Geometry check sheet. Reference: the model listing, model coordinates, mm. Coordinates: 2 decimals unless noted, no trailing zeros. Loops run counter-clockwise (first coordinate to the right, second up) from the corner with the lowest first, then second, coordinate; pieces in that order, holes last. Notation, with made-up numbers: M 61.25,89.25 L 78.25,89.25 A18 ccw 78.25,107.25 Z; hole C 29.5,40 d11. An arc over 180 degrees is marked long. Use CSV: the item, a comma, the result in double quotes.
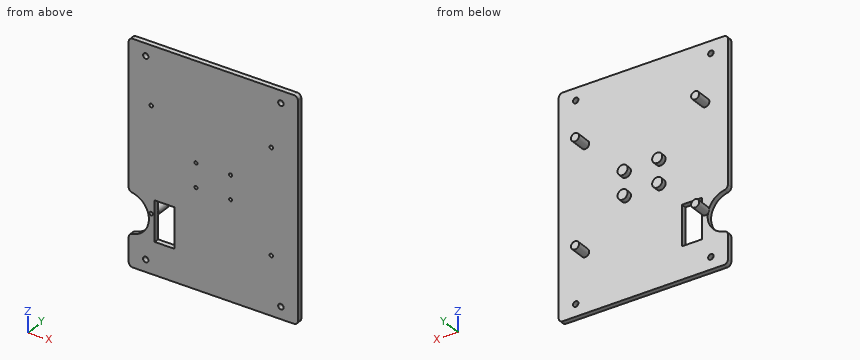
```python
from build123d import *

# Parameters (mm, degrees)
SKETCH1_W           = 107.315
SKETCH1_H           = 139.7
SKETCH1_R           = 1.7272
BOSS_EXTRUDE1_DEPTH = 3.2004
SKETCH2_W           = 12.7
SKETCH2_H           = 25.4
CUT_EXTRUDE1_DEPTH  = 3.2004
SKETCH3_R           = 1.1303
CUT_EXTRUDE2_DEPTH  = 3.2004
FILLET1_R           = 2.54
SKETCH4_R           = 1.02489
CUT_EXTRUDE3_DEPTH  = 3.2004
SKETCH5_R           = 2.54
BOSS_EXTRUDE2_DEPTH = 9.525
SKETCH6_R           = 3.175
BOSS_EXTRUDE3_DEPTH = 3.2004


with BuildPart() as part:
    # Sketch1 → Boss-Extrude1 (new body)
    with BuildSketch(Plane(origin=(0, 0, 0), x_dir=(1, 0, 0), z_dir=(0, 1, 0))):
        with Locations((53.6575, 69.85)):
            Rectangle(SKETCH1_W, SKETCH1_H)
        with Locations((10.795, 132.0165)):
            Circle(SKETCH1_R, mode=Mode.SUBTRACT)
        with Locations((96.52, 132.0165)):
            Circle(SKETCH1_R, mode=Mode.SUBTRACT)
        with Locations((96.52, 7.6835)):
            Circle(SKETCH1_R, mode=Mode.SUBTRACT)
        with Locations((10.795, 7.6835)):
            Circle(SKETCH1_R, mode=Mode.SUBTRACT)
    extrude(amount=BOSS_EXTRUDE1_DEPTH)

    # Sketch2 → Cut-Extrude1 (cut)
    with BuildSketch(Plane(origin=(0, 3.2004, 0), x_dir=(1, 0, 0), z_dir=(0, 1, 0))):
        with Locations((22.86, 106.68)):
            Rectangle(SKETCH2_W, SKETCH2_H)
        with BuildLine():
            Line((0, 119.505365836), (0, 93.854634164))
            ThreePointArc((0, 93.854634164), (12.825365836, 106.68), (0, 119.505365836))
        make_face()
    extrude(amount=-CUT_EXTRUDE1_DEPTH, mode=Mode.SUBTRACT)

    # Sketch3 → Cut-Extrude2 (cut)
    with BuildSketch(Plane(origin=(0, 3.2004, 0), x_dir=(1, 0, 0), z_dir=(0, 1, 0))):
        with Locations((90.4875, 102.87)):
            Circle(SKETCH3_R)
        with Locations((90.4875, 36.83)):
            Circle(SKETCH3_R)
        with Locations((14.2875, 36.83)):
            Circle(SKETCH3_R)
        with Locations((14.2875, 102.87)):
            Circle(SKETCH3_R)
    extrude(amount=-CUT_EXTRUDE2_DEPTH, mode=Mode.SUBTRACT)

    # Fillet1
    fillet1_edges = [part.edges().sort_by_distance(p)[0] for p in [
        (0, 1.6002, -119.505365836),
        (0, 1.6002, -93.854634164),
        (0, 1.6002, -139.7),
        (107.315, 1.6002, -139.7),
        (107.315, 1.6002, 0),
        (0, 1.6002, 0),
    ]]
    fillet(fillet1_edges, radius=FILLET1_R)

    # Sketch4 → Cut-Extrude3 (cut)
    with BuildSketch(Plane(origin=(0, 3.2004, 0), x_dir=(1, 0, 0), z_dir=(0, 1, 0))):
        with Locations((64.6575, 77.35)):
            Circle(SKETCH4_R)
        with Locations((64.6575, 62.35)):
            Circle(SKETCH4_R)
        with Locations((42.6575, 77.35)):
            Circle(SKETCH4_R)
        with Locations((42.6575, 62.35)):
            Circle(SKETCH4_R)
    extrude(amount=-CUT_EXTRUDE3_DEPTH, mode=Mode.SUBTRACT)

    # Sketch5 → Boss-Extrude2 (add)
    with BuildSketch(Plane(origin=(0, 3.2004, 0), x_dir=(1, 0, 0), z_dir=(0, 1, 0))):
        with Locations((90.4875, 102.87)):
            Circle(SKETCH5_R)
        with Locations((90.4875, 36.83)):
            Circle(SKETCH5_R)
        with Locations((14.2875, 36.83)):
            Circle(SKETCH5_R)
        with Locations((14.2875, 102.87)):
            Circle(SKETCH5_R)
    extrude(amount=BOSS_EXTRUDE2_DEPTH)

    # Sketch6 → Boss-Extrude3 (add)
    with BuildSketch(Plane(origin=(0, 3.2004, 0), x_dir=(1, 0, 0), z_dir=(0, 1, 0))):
        with Locations((64.6575, 77.35)):
            Circle(SKETCH6_R)
        with Locations((64.6575, 62.35)):
            Circle(SKETCH6_R)
        with Locations((42.6575, 62.35)):
            Circle(SKETCH6_R)
        with Locations((42.6575, 77.35)):
            Circle(SKETCH6_R)
    extrude(amount=BOSS_EXTRUDE3_DEPTH)


solid = part.part
```
1. Section check C-C, the plane z = -28. Record the cut outline in (x, y) (3 decimals).
The answers:
outline,"M 0,0 L 107.315,0 L 107.315,3.2 L 0,3.2 Z"
2. Section check B-B, the plane y = 9.5. Record the cut outline in (x, z), plus the area to 3 significant figures.
The answers:
outline,"C 14.29,-102.87 d5.08; C 14.29,-36.83 d5.08; C 90.49,-102.87 d5.08; C 90.49,-36.83 d5.08"
area,"81.1 mm^2"
3. Gauge pin test, flat ends, axial feed: P1, Ø2, axis at x = 85, y = 9, coming from the -Z side; P2, Ø2.5, axis at x = 42.66, z = -77.35, coming from the +Y side; P3, Ø1.1, axis at x = 90, z = -103, coming from the -Y side. Record the tip position at first contact, or that the pin passes through.
The answers:
P1,"through"
P2,"y = 6.4"
P3,"y = 3.2"
4. Thickness scan on line 1 (X direction, y = 1.8, z = -36.83) (3 decimals); line 2 (X direction, y = 2.15, z = -77.35) (3 decimals); line 3 (Z direction, x = 96.52, y = 1.1). Record the ranges inside material, lowest first. Write a range as [from, to].
The answers:
line 1,"[0, 13.157], [15.418, 89.357], [91.618, 107.315]"
line 2,"[0, 41.633], [43.682, 63.633], [65.682, 107.315]"
line 3,"[-139.7, -133.74], [-130.29, -9.41], [-5.96, 0]"
5. Section check A-A, the plane x = 96.52. Record the cut outline in (y, z), plus the area to 3 significant figures.
The answers:
outline,"M 0,-139.7 L 3.2,-139.7 L 3.2,-133.74 L 0,-133.74 Z; M 0,-130.29 L 3.2,-130.29 L 3.2,-9.41 L 0,-9.41 Z; M 0,-5.96 L 3.2,-5.96 L 3.2,0 L 0,0 Z"
area,"425 mm^2"
